CAD build for the part. Positions are in the model's coordinates, mm. A direction names the side the tool comes from. Round coordinates to 2 decimals unless told otherwise and drop trailing zeros. Loops run counter-clockwise (first coordinate to the right, second up) from the corner with the lowest first, then second, coordinate; pieces in that order, holes last.
from build123d import *

# Parameters (mm, degrees)
BOSS_EXTRUDE1_DEPTH   = 6.35
F_8_CLEARANCE_HOLE1_D = 4.4958


with BuildPart() as part:
    # Sketch1 → Boss-Extrude1 (new body)
    with BuildSketch(Plane.XY):
        Polygon((40.64, 122.682), (40.64, 94.234), (59.69, 94.234), (59.69, 75.184), (95.1484, 75.184), (95.1484, -81.28), (8.89, -81.28), (8.89, -44.45), (-3.81, -44.45), (-3.81, -12.7), (-26.67, -12.7), (-26.67, 122.682), align=None)
        Polygon((90.0684, 62.484), (27.94, 62.484), (21.59, 62.484), (21.59, 117.602), (-21.59, 117.602), (-21.59, 0), (21.59, 0), (27.94, 0), (27.94, -76.2), (90.0684, -76.2), align=None, mode=Mode.SUBTRACT)
    extrude(amount=BOSS_EXTRUDE1_DEPTH)

    # #8 Clearance Hole1 (through all)
    with Locations(Plane.XY.offset(6.35)):
        with Locations((9.538335251, -23.376368086), (40.402766773, 80.728472273)):
            Hole(F_8_CLEARANCE_HOLE1_D / 2)


solid = part.part
Item 1: Mould opens along Y. For faces 4 (the cylindrical face through (42.187, 79.361, 3.131)), 5 (the flat face through (7, 122.682, 3)), 6 (the flat face through (53, -81.28, 3)), 7 (the flat face through (4, 0, 3)) say: released by +Y, released by -Y, zero draft, split by the parting line, or undercut.
Verdict:
face 4: undercut
face 5: released by +Y
face 6: released by -Y
face 7: undercut
Item 2: Wall check: L1, parallel to X at y = -64.5, z = 5.5; L2, parallel to Y at x = 85, z = 2; L3, parallel to Y at x = 44.5, z = 5.75. Give the ranges that are in metal, low to high.
Verdict:
L1: x = 8.89 to 27.94, 90.07 to 95.15
L2: y = -81.28 to -76.2, 62.48 to 75.18
L3: y = -81.28 to -76.2, 62.48 to 94.23
Item 3: Cut at C-C (z = 5). List the corners of the cut face in (x, y).
Verdict:
outline: (-26.67, -12.7) - (-3.81, -12.7) - (-3.81, -44.45) - (8.89, -44.45) - (8.89, -81.28) - (95.15, -81.28) - (95.15, 75.18) - (59.69, 75.18) - (59.69, 94.23) - (40.64, 94.23) - (40.64, 122.68) - (-26.67, 122.68) - close; hole (-21.59, 0) - (27.94, 0) - (27.94, -76.2) - (90.07, -76.2) - (90.07, 62.48) - (21.59, 62.48) - (21.59, 117.6) - (-21.59, 117.6) - close; hole circle Ø4.5 at (9.54, -23.38); hole circle Ø4.5 at (40.4, 80.73)
Item 4: Cut at A-A (y = -65.5). List the corners of the cut face in (x, z), plus the area to 3 significant figures.
Verdict:
outline: (8.89, 0) - (27.94, 0) - (27.94, 6.35) - (8.89, 6.35) - close; (90.07, 0) - (95.15, 0) - (95.15, 6.35) - (90.07, 6.35) - close
area: 153 mm2
Item 5: Flat gauge pins, fed straight in: P1, Ø3, axis at x = 3.5, z = 2, coming from the -Y side; P2, Ø1.9, axis at y = 105, z = 1.5, coming from the +X side; P3, Ø3, axis at x = 54, z = 5.5, coming from the +Y side. Where does each tip first touch, or does it go through?
Verdict:
P1: stops at y = -44.45
P2: stops at x = 40.64
P3: stops at y = 94.23
Item 6: Cut at B-B (x = 1). List the corners of the cut face in (y, z), plus the area to 3 significant figures.
Verdict:
outline: (-44.45, 0) - (0, 0) - (0, 6.35) - (-44.45, 6.35) - close; (117.6, 0) - (122.68, 0) - (122.68, 6.35) - (117.6, 6.35) - close
area: 315 mm2
Item 7: 3-axis set-ups, long thin cutter, end or side, ignore diameter. For faces 1 (the flat face through (-3.81, -29, 3)), 2 (the flat face through (77, 75.184, 3)), 3 (the flat face through (59, -76.2, 3)): which of +Z, -Z, +X, -X, +Y, -Y reach the whole face in a straight line?
Verdict:
face 1: +Z, -Z, -X, -Y
face 2: +Z, -Z, +X, +Y
face 3: +Z, -Z
